from build123d import *

# Parameters (mm, degrees)
SKETCH_1_W      = 101
SKETCH_1_H      = 46
SKETCH_1_W_2    = 97
SKETCH_1_H_2    = 33
EXTRUDE_1_DEPTH = 2
FILLET_1_R      = 1
FILLET_2_R      = 1


with BuildPart() as part:
    # 草图1 → 凸台-拉伸1 (new body)
    with BuildSketch(Plane.XY):
        Rectangle(SKETCH_1_W, SKETCH_1_H)
        with Locations((0, -2.5)):
            Rectangle(SKETCH_1_W_2, SKETCH_1_H_2, mode=Mode.SUBTRACT)
    extrude(amount=EXTRUDE_1_DEPTH)

    # 圆角1
    fillet_1_edges = [part.edges().sort_by_distance(p)[0] for p in [
        (-50.5, 23, 1),
    ]]
    fillet(fillet_1_edges, radius=FILLET_1_R)

    # 圆角2
    fillet_2_edges = [part.edges().sort_by_distance(p)[0] for p in [
        (50.5, -23, 1),
        (-50.5, -23, 1),
        (50.5, 23, 1),
    ]]
    fillet(fillet_2_edges, radius=FILLET_2_R)


solid = part.part
The listing builds one solid part. Answer for the finished solid, in the listing's coordinates (mm). A direction names the side the tool comes from. Round coordinates to 2 decimals unless told otherwise and drop trailing zeros. Write each loop counter-clockwise with the first axis right and the second up, starting at its lowest first coordinate (ties: lowest second). Pieces come first, ordered by that corner, then holes. Notation, with made-up numbers: (78, 31) - (87, 31) arc R21 cw to (87, 35) - close; hole circle Ø9 at (-7.75, 35). An arc over 180 degrees is marked (long way). Use a Markdown table: item, result. Add a question column.
1. The part is cut by section C-C (y = -3.5). Write down the section's boundary in (x, z), and give its area (3 significant figures).
2. The part is cut by section B-B (z = 1.05). Write down the section's boundary in (x, y).
3. A flat-ended cylindrical pin translates along its axis: P1, Ø12, axis at x = -33.5, y = 13, coming from the +Z side. Find the tip coordinate at first contact, or state that the pin passes through.
4. A tool of negligible diameter and unlimited length cuts with its end or side. For faces 5 (the face through (-1, 14, 1)), 6 (the face through (-4, 17, 2)), from which of +Z, -Z, +X, -X, +Y, -Y can it reach the whole face along a straight path? Write none if from no direction.
5. For a pull along X with two mould halves and no side action, classify faces 1 (the face through (-4, 17, 0)), 2 (the face through (48.5, -3, 1)), 3 (the face through (50.5, 0, 1)), 4 (the face through (-48.5, -3, 1)) as +X half, -X half, draft (parallel to the pull), parting line (faces both ways), or undercut.
6. Consider line 1 (Y direction, x = -14.5, z = 0.3); line 2 (X direction, y = -1, z = 1.05). Determine where each line is inside the solid, lowest interval first.
7. The part is cut by section A-A (x = 11.5). Write down the section's boundary in (y, z), and give its area (3 significant figures).
Reported:
| question | item | result |
|---|---|---|
| 1 | outline | (-50.5, 0) - (-48.5, 0) - (-48.5, 2) - (-50.5, 2) - close; (48.5, 0) - (50.5, 0) - (50.5, 2) - (48.5, 2) - close |
| 1 | area | 8.00 mm^2 |
| 2 | outline | (-50.5, -22) arc R1 ccw to (-49.5, -23) - (49.5, -23) arc R1 ccw to (50.5, -22) - (50.5, 22) arc R1 ccw to (49.5, 23) - (-49.5, 23) arc R1 ccw to (-50.5, 22) - close; hole (-48.5, -19) - (48.5, -19) - (48.5, 14) - (-48.5, 14) - close |
| 3 | P1 | z = 2 |
| 4 | face 5 | +Z, -Z |
| 4 | face 6 | +Z, +X, -X, +Y, -Y |
| 5 | face 1 | draft |
| 5 | face 2 | undercut |
| 5 | face 3 | +X half |
| 5 | face 4 | undercut |
| 6 | line 1 | -23 to -19, 14 to 23 |
| 6 | line 2 | -50.5 to -48.5, 48.5 to 50.5 |
| 7 | outline | (-23, 0) - (-19, 0) - (-19, 2) - (-23, 2) - close; (14, 0) - (23, 0) - (23, 2) - (14, 2) - close |
| 7 | area | 26.0 mm^2 |
